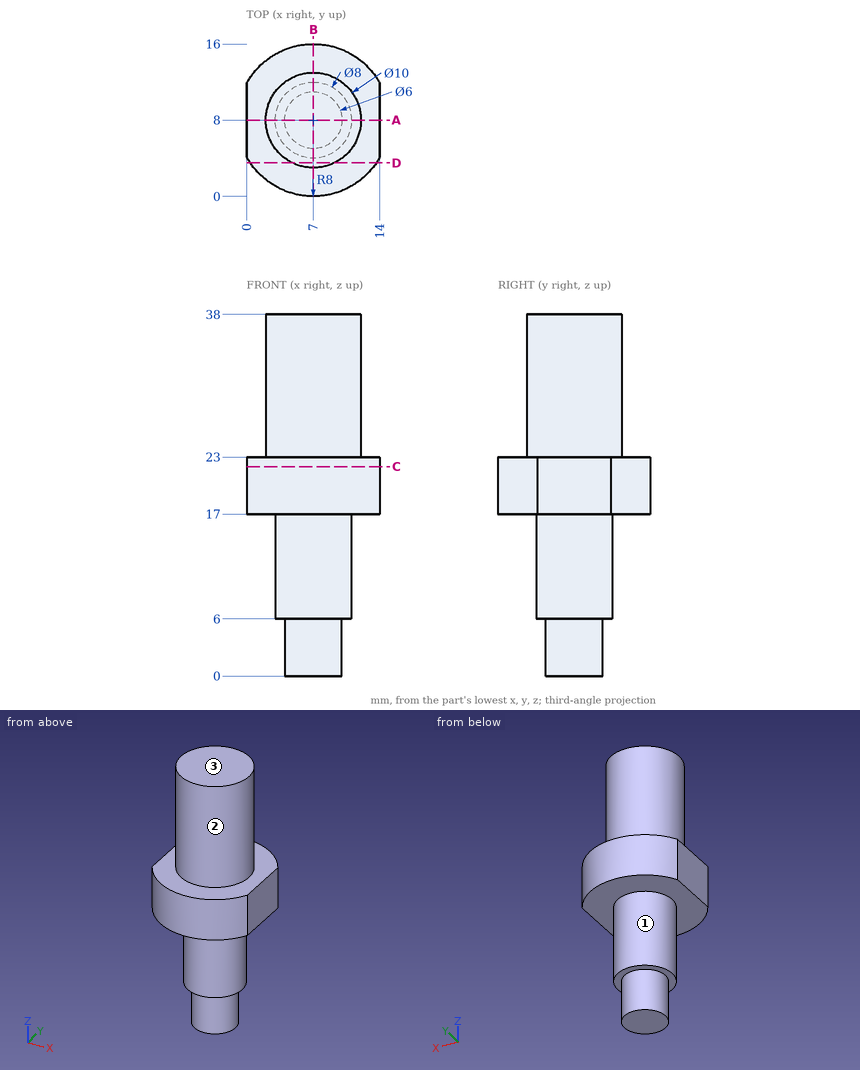
Study the drawing (mm; zero at the part's minimum x, y, z) and answer. A direction names the side the tool comes from. Round coordinates to 2 decimals unless told otherwise and drop trailing zeros. Order: outer loops, then holes, each group sorted by start corner. A loop starts at its lowest first (then second) coordinate and runs counter-clockwise, first axis right, second up. Notation, with made-up numbers: (70.5, -26) -> (125.5, -26) arc R12 cw to (125.5, -22) -> close; hole circle Ø7 at (-35.75, -24). An arc over 180 degrees is marked (long way). Answer as CSV lines item,"result". Start each with the question number.
(1) The part is cut by section C-C (z = 22). Determine the outline of the cut face in (x, y), then the cut area to 3 significant figures.
(2) A tool of negligible diameter and unlimited length cuts with its end or side. For the marked faces 1, 2 and 3, from which of +Z, -Z, +X, -X, +Y, -Y can it reach the whole face along a straight path? Write none if from no direction.
(3) The part is cut by section D-D (y = 3.5). Determine the outline of the cut face in (x, z), then the cut area to 3 significant figures.
(4) Flat-ended cylindrical pins translate along their axes: pin 1 Ø1 at (y, z) = (8, 11.5) entering from +X; pin 2 Ø3 at (y, z) = (13.5, 34) entering from -X; pin 3 Ø8 at (x, z) = (3, 11.5) entering from +Y. Find the tip coordinate at first contact, or state that the pin passes through.
(5) The part is cut by section A-A (y = 8). Determine the outline of the cut face in (x, z), then the cut area to 3 significant figures.
(6) Find the intervals of material crossed by probe 1 along Y at (x, z) = (7, 5.5); probe 2 along Z at (x, y) = (9, 13.75); probe 3 along Z at (x, y) = (10.5, 10.75), in increasing order. Write a range as from..to.
(7) The part is cut by section B-B (x = 7). Determine the outline of the cut face in (y, z).
Evaluation:
1,outline,"(0, 4.13) arc R8 ccw to (14, 4.13) -> (14, 11.87) arc R8 ccw to (0, 11.87) -> close"
1,area,"191 mm²"
2,face 1,"-Z"
2,face 2,"+Z"
2,face 3,"+Z, +X, -X, +Y, -Y"
3,outline,"(0.39, 17) -> (13.61, 17) -> (13.61, 23) -> (9.18, 23) -> (9.18, 38) -> (4.82, 38) -> (4.82, 23) -> (0.39, 23) -> close"
3,area,"145 mm²"
4,pin 1,"x = 11"
4,pin 2,"x = 4"
4,pin 3,"y = 12"
5,outline,"(0, 17) -> (3, 17) -> (3, 6) -> (4, 6) -> (4, 0) -> (10, 0) -> (10, 6) -> (11, 6) -> (11, 17) -> (14, 17) -> (14, 23) -> (12, 23) -> (12, 38) -> (2, 38) -> (2, 23) -> (0, 23) -> close"
5,area,"358 mm²"
6,probe 1,"5..11"
6,probe 2,"17..23"
6,probe 3,"17..38"
7,outline,"(0, 17) -> (4, 17) -> (4, 6) -> (5, 6) -> (5, 0) -> (11, 0) -> (11, 6) -> (12, 6) -> (12, 17) -> (16, 17) -> (16, 23) -> (13, 23) -> (13, 38) -> (3, 38) -> (3, 23) -> (0, 23) -> close"
